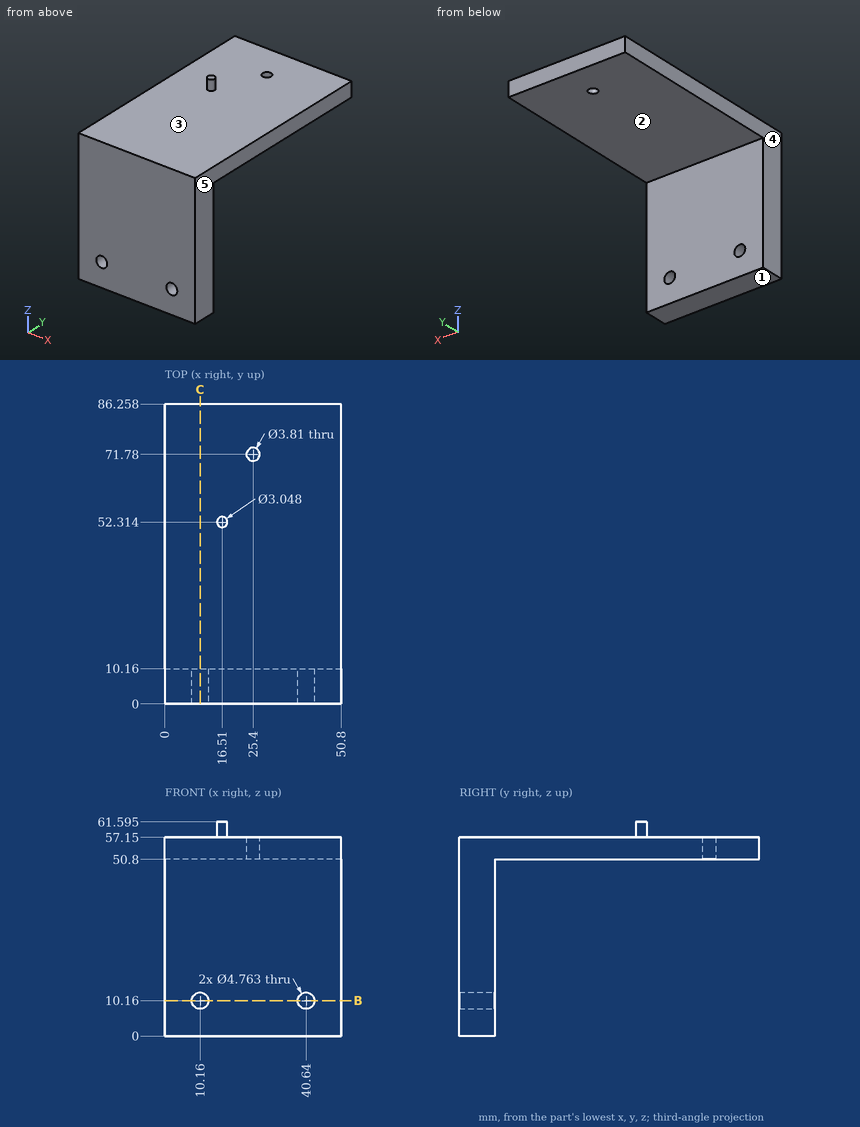
Design review of the part shown in the three views and the two pictorial views. Dimensions are in mm from the part's minimum x, y and z. A direction names the side the tool comes from. Give positions to 0.01 mm unless a question says otherwise; leave off trailing zeros. Loops run counter-clockwise (first coordinate to the right, second up) from the corner with the lowest first, then second, coordinate; pieces in that order, holes last. Notation, with made-up numbers: (12, -36.5) -> (69, -36.5) arc R16 ccw to (69, -25.5) -> close; hole circle Ø10 at (55, -20). An arc over 180 degrees is marked (long way). Put each result on its own line as item: value. Start each with the question number.
1. Mouldability with a two-part tool opening along X and no side actions: class the marked faces 3, 4 and 5 as released by +X, released by -X, zero draft, split by the parting line, or undercut.
2. Wall thickness on probe 1 along X at (y, z) = (3, 10.16); probe 2 along Z at (x, y) = (40.64, 4.5); probe 3 along Z at (x, y) = (38.5, 61): over which ranges is each line inside the solid? List them lowest first.
3. We need section B-B on z = 10.16. State the section outline as (x, y) points.
4. We need section C-C on x = 10.16. State the section outline as (y, z) points.
5. For the marked faces 1 and 2, list the 3-axis set-ups (+Z, -Z, +X, -X, +Y, -Y) from which the entire face can be reached by the end or side of a thin tool; tool diameter is ignored.
6. Clearance check with flat-ended pins moving along their axes: P1, Ø10, axis at x = 29.5, z = 44.5, coming from the -Y side; P2, Ø5.5, axis at x = 40.64, z = 10.16, coming from the +Y side; P3, Ø3, axis at x = 15, y = 23, coming from the +Z side; P4, Ø12, axis at x = 8, y = 65.5, coming from the -Z side. State where each tip first meets the part, or that it passes through.
Determined:
1. face 3: zero draft
1. face 4: released by -X
1. face 5: released by +X
2. probe 1: 0 to 7.78, 12.54 to 38.26, 43.02 to 50.8
2. probe 2: 0 to 7.78, 12.54 to 57.15
2. probe 3: 50.8 to 57.15
3. outline: (0, 0) -> (7.78, 0) -> (7.78, 10.16) -> (0, 10.16) -> close; (12.54, 0) -> (38.26, 0) -> (38.26, 10.16) -> (12.54, 10.16) -> close; (43.02, 0) -> (50.8, 0) -> (50.8, 10.16) -> (43.02, 10.16) -> close
4. outline: (0, 0) -> (10.16, 0) -> (10.16, 7.78) -> (0, 7.78) -> close; (0, 12.54) -> (10.16, 12.54) -> (10.16, 50.8) -> (86.26, 50.8) -> (86.26, 57.15) -> (0, 57.15) -> close
5. face 1: -Z, +X, -X, +Y, -Y
5. face 2: -Z, +X, -X, +Y
6. P1: y = 0
6. P2: y = 10.16
6. P3: z = 57.15
6. P4: z = 50.8
